For this review, take the finished solid that the model builds, in its own axes (mm). Round coordinates to 2 decimals unless told otherwise and drop trailing zeros. Order: outer loops, then holes, each group sorted by start corner. A loop starts at its lowest first (then second) coordinate and runs counter-clockwise, first axis right, second up. Notation, with made-up numbers: (86.5, 63.5) -> (117.5, 63.5) arc R10 cw to (117.5, 77.5) -> close; hole circle Ø9 at (-28, 5). An arc over 180 degrees is marked (long way). Use a Markdown table: item, result. Add a question column.
1) Consider section A-A (z = 14.75). State the section outline as (x, y) points.
2) Consider section B-B (x = 58). State the section outline as (y, z) points, plus the area to 3 significant figures.
3) Consider section D-D (x = 236.5). State the section outline as (y, z) points.
4) Wall thickness on line 1 along Y through (x, z) = (25, 17); line 2 along Z through (x, y) = (298, 80): over which ranges is each line inside the solid? List them lowest first. Write a range as [from, to].
5) Clearance check with flat-ended pins moving along their axes: P1, Ø3, axis at x = 227, y = 329, coming from the +Z side; P2, Ø1.5, axis at y = 55, z = 12, coming from the -X side. State where each tip first meets the part, or that it passes through.
```python
from build123d import *

# Parameters (mm, degrees)
SKETCH_W     = 400
SKETCH_H     = 400
PAD_DEPTH    = 2
SKETCH001_R  = 14
PAD001_DEPTH = 30
SKETCH002_R  = 13
HOLE_DEPTH   = 30


with BuildPart() as part:
    # Sketch → Pad (new body)
    with BuildSketch(Plane.XY):
        with Locations((200, 200)):
            Rectangle(SKETCH_W, SKETCH_H)
    extrude(amount=PAD_DEPTH)

    # Sketch001 → Pad001 (join)
    with BuildSketch(Plane.XY):
        with Locations((25, 25)):
            Circle(SKETCH001_R)
        with Locations((58, 25)):
            Circle(SKETCH001_R)
        with Locations((58, 58)):
            Circle(SKETCH001_R)
        with Locations((25, 58)):
            Circle(SKETCH001_R)
    extrude(amount=PAD001_DEPTH)

    # Sketch002 → Hole (cut)
    with BuildSketch(Plane.XY):
        with Locations((25, 58)):
            Circle(SKETCH002_R)
        with Locations((58, 58)):
            Circle(SKETCH002_R)
        with Locations((58, 25)):
            Circle(SKETCH002_R)
        with Locations((25, 25)):
            Circle(SKETCH002_R)
    extrude(amount=HOLE_DEPTH, mode=Mode.SUBTRACT)


solid = part.part
```
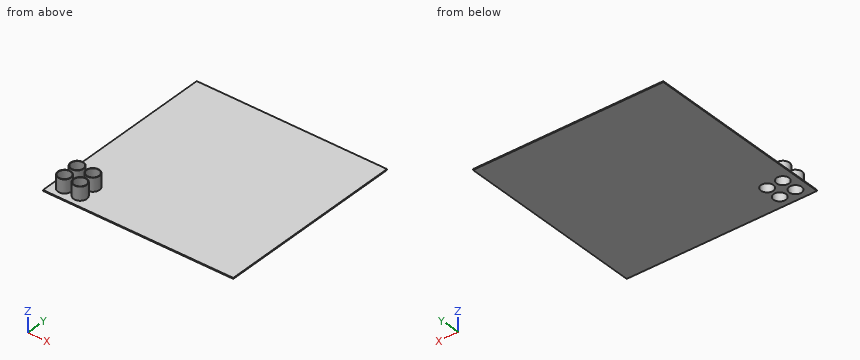
Results list:
| question | item | result |
|---|---|---|
| 1 | outline | circle Ø28 at (25, 25); circle Ø28 at (25, 58); circle Ø28 at (58, 25); circle Ø28 at (58, 58); hole circle Ø26 at (25, 25); hole circle Ø26 at (25, 58); hole circle Ø26 at (58, 25); hole circle Ø26 at (58, 58) |
| 2 | outline | (0, 0) -> (12, 0) -> (12, 30) -> (11, 30) -> (11, 2) -> (0, 2) -> close; (38, 0) -> (45, 0) -> (45, 30) -> (44, 30) -> (44, 2) -> (39, 2) -> (39, 30) -> (38, 30) -> close; (71, 0) -> (400, 0) -> (400, 2) -> (72, 2) -> (72, 30) -> (71, 30) -> close |
| 2 | area | 808 mm2 |
| 3 | outline | (0, 0) -> (400, 0) -> (400, 2) -> (0, 2) -> close |
| 4 | line 1 | [11, 12], [38, 39], [44, 45], [71, 72] |
| 4 | line 2 | [0, 2] |
| 5 | P1 | z = 2 |
| 5 | P2 | x = 11.18 |
